Verification items for the finished model (mm, model axes). A direction names the side the tool comes from. Round coordinates to 2 decimals unless told otherwise and drop trailing zeros. Write each loop counter-clockwise with the first axis right and the second up, starting at its lowest first coordinate (ties: lowest second). Pieces come first, ordered by that corner, then holes. Notation, with made-up numbers: M -20,52.5 L 25,52.5 A22 ccw 25,83.5 Z; hole C -19.5,46.25 d4. An arc over 180 degrees is marked long. Use a Markdown table: item, result. Add a question column.
from build123d import *

# Parameters (mm, degrees)
BOSS_EXTRUDE1_DEPTH = 2.38125
SKETCH2_R           = 3.175
BOSS_EXTRUDE2_DEPTH = 11.1125


with BuildPart() as part:
    # Sketch1 → Boss-Extrude1 (new, symmetric)
    with BuildSketch(Plane(origin=(0, 0, 0), x_dir=(1, 0, 0), z_dir=(0, 1, 0))):
        Polygon((0, 8.248891971), (-7.14375, 4.124445986), (-7.14375, -4.124445986), (0, -8.248891971), (7.14375, -4.124445986), (7.14375, 4.124445986), align=None)
    extrude(amount=BOSS_EXTRUDE1_DEPTH, both=True)

    # Sketch2 → Boss-Extrude2 (add)
    with BuildSketch(Plane(origin=(0, 2.38125, 0), x_dir=(1, 0, 0), z_dir=(0, 1, 0))):
        with Locations(Location((0, 0, 0), (0, 0, 270))):
            Circle(SKETCH2_R)
    extrude(amount=BOSS_EXTRUDE2_DEPTH)


solid = part.part
1. Cross-section at D-D on y = 11. Enter the section's corners in (x, z) (3 decimals), plus the area to 3 significant figures.
2. Cross-section at C-C on x = -4.75. Enter the section's corners in (y, z), plus the area to 3 significant figures.
3. Depth check by flat-ended pin: pin 1 Ø3 at (x, y) = (-2.5, 0) entering from -Z; pin 2 Ø1 at (y, z) = (6.5, -3) entering from +X; pin 3 Ø8 at (y, z) = (3, -2.5) entering from +X. Enter the tip coordinate at first touch or a pass-through.
4. Scan lines: line 1 along Y through (x, z) = (-5, 3.75); line 2 along X through (y, z) = (12.25, 0) (3 decimals); line 3 along Z through (x, y) = (2.75, 12.25). Record each from-to range of solid material in increasing order. Write a range as from..to.
5. Cross-section at A-A on z = 0. Enter the section's corners in (x, y) (3 decimals).
6. Access from +Z, -Z, +X, -X, +Y, -Y to the whole of each face (thin tool, end or side, straight path). Record for faces 1 (the flat face through (0, 2.381, 4)), 2 (the flat face through (3.62, 0.03, -6.16)).
7. Cross-section at B-B on y = -1.5. Enter the section's corners in (x, z).
Answer:
| question | item | result |
|---|---|---|
| 1 | outline | C 0,0 d6.35 |
| 1 | area | 31.7 mm^2 |
| 2 | outline | M -2.38,-5.51 L 2.38,-5.51 L 2.38,5.51 L -2.38,5.51 Z |
| 2 | area | 52.4 mm^2 |
| 3 | pin 1 | stops at z = -7.67 |
| 3 | pin 2 | stops at x = 1.96 |
| 3 | pin 3 | stops at x = 7.14 |
| 4 | line 1 | y = -2.38..2.38 |
| 4 | line 2 | x = -3.175..3.175 |
| 4 | line 3 | z = -1.59..1.59 |
| 5 | outline | M -7.144,-2.381 L 7.144,-2.381 L 7.144,2.381 L 3.175,2.381 L 3.175,13.494 L -3.175,13.494 L -3.175,2.381 L -7.144,2.381 Z |
| 6 | face 1 | +Y |
| 6 | face 2 | -Z, +X, +Y, -Y |
| 7 | outline | M -7.14,-4.12 L 0,-8.25 L 7.14,-4.12 L 7.14,4.12 L 0,8.25 L -7.14,4.12 Z |
